Read the model definition and answer for the solid it produces. Units are mm, in the model's axes. Face numbers are marked on the shaded views. A direction names the side the tool comes from. Coordinates: 2 decimals unless noted, no trailing zeros. Order: outer loops, then holes, each group sorted by start corner. A loop starts at its lowest first (then second) coordinate and runs counter-clockwise, first axis right, second up. Notation, with made-up numbers: (-21.75, -10) - (-11.75, -10) arc R13 ccw to (-11.75, 2) - close; hole circle Ø1 at (55.5, 38). An arc over 180 degrees is marked (long way). Write item = value, one per line.
from build123d import *

# Parameters (mm, degrees)
AUFSATZ_LINEAR_AUSTRAGEN1_DEPTH = 3
F_4_0_4_DURCHMESSER_BOHRUNG1_D  = 4
SCHNITT_LINEAR_AUSTRAGEN1_DEPTH = 3
VERRUNDUNG2_R                   = 2


with BuildPart() as part:
    # Skizze1 → Aufsatz-Linear austragen1 (new body)
    with BuildSketch(Plane.XY):
        Polygon((-11, 5), (-11, 0), (11, 0), (11, 5), (5, 5), (5, 9), (11, 9), (11, 19), (-11, 19), (-11, 9), (-5, 9), (-5, 5), align=None)
    extrude(amount=AUFSATZ_LINEAR_AUSTRAGEN1_DEPTH)

    # Ø4.0 (4) Durchmesser Bohrung1 (through all)
    with Locations(Plane.XY.offset(3)):
        with Locations((7, 15)):
            Hole(F_4_0_4_DURCHMESSER_BOHRUNG1_D / 2)

    # Skizze4 → Schnitt-Linear austragen1 (cut)
    with BuildSketch(Plane.XY.offset(3)):
        Polygon((-11, 14), (0.509428342, 19), (-11, 19), align=None)
    extrude(amount=-SCHNITT_LINEAR_AUSTRAGEN1_DEPTH, mode=Mode.SUBTRACT)

    # Verrundung2
    verrundung2_edges = [part.edges().sort_by_distance(p)[0] for p in [
        (11, 19, 1.5),
        (11, 0, 1.5),
        (-11, 0, 1.5),
        (-11, 14, 1.5),
        (0.509428342, 19, 1.5),
    ]]
    fillet(verrundung2_edges, radius=VERRUNDUNG2_R)


solid = part.part
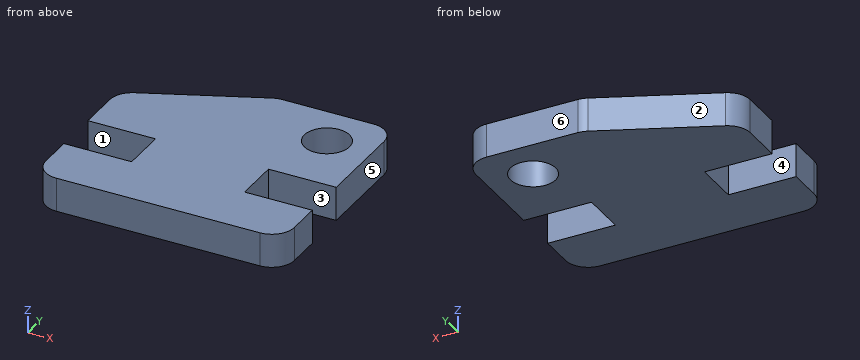
1) The part is cut by section D-D (y = 8.25). Determine the outline of the cut face in (x, z), and give its area (3 significant figures).
Returned:
outline = (-5, 0) - (5, 0) - (5, 3) - (-5, 3) - close
area = 30.0 mm^2
2) The part is cut by section B-B (z = 1.5). Determine the outline of the cut face in (x, y).
Returned:
outline = (-11, 2) arc R2 ccw to (-9, 0) - (9, 0) arc R2 ccw to (11, 2) - (11, 5) - (5, 5) - (5, 9) - (11, 9) - (11, 17) arc R2 ccw to (9, 19) - (0.93, 19) arc R2 ccw to (0.13, 18.83) - (-9.8, 14.52) arc R2 ccw to (-11, 12.69) - (-11, 9) - (-5, 9) - (-5, 5) - (-11, 5) - close; hole circle Ø4 at (7, 15)
3) Straight lines are drawn through the part: line 1 along Y through (x, z) = (7, 2.3); line 2 along Y through (x, z) = (6.25, 2.65); line 3 along X through (y, z) = (7.25, 0.45). For each, find the intervals that lie inside material, in ascending order. Write a range as from..to.
Returned:
line_1 = 0..5, 9..13, 17..19
line_2 = 0..5, 9..13.15, 16.85..19
line_3 = -5..5
4) The part is cut by section C-C (y = 15). Determine the outline of the cut face in (x, z).
Returned:
outline = (-8.7, 0) - (5, 0) - (5, 3) - (-8.7, 3) - close; (9, 0) - (11, 0) - (11, 3) - (9, 3) - close
5) The part is cut by section A-A (x = 7). Determine the outline of the cut face in (y, z).
Returned:
outline = (0, 0) - (5, 0) - (5, 3) - (0, 3) - close; (9, 0) - (13, 0) - (13, 3) - (9, 3) - close; (17, 0) - (19, 0) - (19, 3) - (17, 3) - close
6) Flat-ended cylindrical pins translate along their axes: pin 1 Ø1.5 at (y, z) = (8, 1.5) entering from +X; pin 2 Ø3 at (x, y) = (-6, 4) entering from -Z; pin 3 Ø3 at (x, y) = (7, 7) entering from +Z. Find the tip coordinate at first contact, or state that the pin passes through.
Returned:
pin_1 = 5
pin_2 = 0
pin_3 = through
7) Determine the mould class of the marked faces 4, 5 and 6 for opening direction Y: pulls with the +Y half, pulls with the -Y half, needs draft (parallel to the pull), parting line crosses it, or undercut.
Returned:
face_4 = undercut
face_5 = needs draft
face_6 = pulls with the +Y half
8) For the marked faces 1, 2 and 3, determine the directions among +Z, -Z, +X, -X, +Y, -Y from which every point of the face is accessible in a straight line to the end or side of a thin tool.
Returned:
face_1 = +Z, -Z, -X
face_2 = +Z, -Z, -X, +Y
face_3 = +Z, -Z, +X
